from build123d import *

# Parameters (mm, degrees)
SKETCH6_W                    = 35
SKETCH6_H                    = 40
BASE_FLANGE2_DEPTH           = 1.4
EDGE_FLANGE1_STRIP_W         = 11.6
EDGE_FLANGE1_STRIP_H         = 1.4
EDGE_FLANGE1_STRIP_CUT_DEPTH = 40
EDGE_FLANGE1_DEPTH           = 40
EDGE_FLANGE2_STRIP_W         = 11.6
EDGE_FLANGE2_STRIP_H         = 1.4
EDGE_FLANGE2_STRIP_CUT_DEPTH = 40
EDGE_FLANGE2_DEPTH           = 40
EDGE_FLANGE3_STRIP_W         = 11.6
EDGE_FLANGE3_STRIP_H         = 1.4
EDGE_FLANGE3_STRIP_CUT_DEPTH = 40
EDGE_FLANGE3_DEPTH           = 40
EDGE_FLANGE4_STRIP_W         = 11.6
EDGE_FLANGE4_STRIP_H         = 1.4
EDGE_FLANGE4_STRIP_CUT_DEPTH = 40
EDGE_FLANGE4_DEPTH           = 40
CUT_EXTRUDE2_DEPTH           = 76.623541308
CUT_EXTRUDE2_DEPTH_BACK      = 76.623541308
SKETCH11_R                   = 7.5
SKETCH11_R_2                 = 1.7
CUT_EXTRUDE3_DEPTH           = 76.795514379
CUT_EXTRUDE3_DEPTH_BACK      = 76.795514379
SKETCH26_R                   = 1.7
CUT_EXTRUDE4_DEPTH           = 76.795514379
CUT_EXTRUDE4_DEPTH_BACK      = 76.795514379
SKETCH27_R                   = 1.7


# Sheet-metal steps are written as plain solids
with BuildPart() as part:
    # Sketch6 → Base-Flange2 (new body)
    with BuildSketch(Plane.XY):
        with Locations((17.5, 20)):
            Rectangle(SKETCH6_W, SKETCH6_H)
    extrude(amount=-BASE_FLANGE2_DEPTH)

    # Edge-Flange1 strip (across the edge) → Edge-Flange1 strip cut (cut)
    with BuildSketch(Plane.XZ.offset(-40)):
        with Locations((-1.4, -0.7)):
            Rectangle(EDGE_FLANGE1_STRIP_W, EDGE_FLANGE1_STRIP_H)
    extrude(amount=EDGE_FLANGE1_STRIP_CUT_DEPTH, mode=Mode.SUBTRACT)

    # Edge-Flange1 section (across the edge) → Edge-Flange1 (add)
    with BuildSketch(Plane.XZ.offset(-40)):
        with BuildLine():
            Line((0, 3), (0, 8.6))
            Line((0, 8.6), (1.4, 8.6))
            Line((1.4, 8.6), (1.4, 3))
            ThreePointArc((1.4, 3), (2.278679656, 0.878679656), (4.4, 0))
            Line((4.4, 0), (4.4, -1.4))
            ThreePointArc((4.4, -1.4), (1.288730163, -0.111269837), (0, 3))
        make_face()
    extrude(amount=EDGE_FLANGE1_DEPTH)

    # Edge-Flange2 strip (across the edge) → Edge-Flange2 strip cut (cut)
    with BuildSketch(Plane(origin=(35, 0, 0), x_dir=(-1, 0, 0), z_dir=(0, 1, 0))):
        with Locations((-1.4, -0.7)):
            Rectangle(EDGE_FLANGE2_STRIP_W, EDGE_FLANGE2_STRIP_H)
    extrude(amount=EDGE_FLANGE2_STRIP_CUT_DEPTH, mode=Mode.SUBTRACT)

    # Edge-Flange2 section (across the edge) → Edge-Flange2 (add)
    with BuildSketch(Plane(origin=(35, 0, 0), x_dir=(-1, 0, 0), z_dir=(0, 1, 0))):
        with BuildLine():
            Line((0, 3), (0, 8.6))
            Line((0, 8.6), (1.4, 8.6))
            Line((1.4, 8.6), (1.4, 3))
            ThreePointArc((1.4, 3), (2.278679656, 0.878679656), (4.4, 0))
            Line((4.4, 0), (4.4, -1.4))
            ThreePointArc((4.4, -1.4), (1.288730163, -0.111269837), (0, 3))
        make_face()
    extrude(amount=EDGE_FLANGE2_DEPTH)

    # Edge-Flange3 strip (across the edge) → Edge-Flange3 strip cut (cut)
    with BuildSketch(Plane(origin=(0, 0, 8.6), x_dir=(0, 0, -1), z_dir=(0, 1, 0))):
        with Locations((-1.4, -0.7)):
            Rectangle(EDGE_FLANGE3_STRIP_W, EDGE_FLANGE3_STRIP_H)
    extrude(amount=EDGE_FLANGE3_STRIP_CUT_DEPTH, mode=Mode.SUBTRACT)

    # Edge-Flange3 section (across the edge) → Edge-Flange3 (add)
    with BuildSketch(Plane(origin=(0, 0, 8.6), x_dir=(0, 0, -1), z_dir=(0, 1, 0))):
        with BuildLine():
            Line((0, 3), (0, 28.6))
            Line((0, 28.6), (1.4, 28.6))
            Line((1.4, 28.6), (1.4, 3))
            ThreePointArc((1.4, 3), (2.278679656, 0.878679656), (4.4, 0))
            Line((4.4, 0), (4.4, -1.4))
            ThreePointArc((4.4, -1.4), (1.288730163, -0.111269837), (0, 3))
        make_face()
    extrude(amount=EDGE_FLANGE3_DEPTH)

    # Edge-Flange4 strip (across the edge) → Edge-Flange4 strip cut (cut)
    with BuildSketch(Plane(origin=(35, 40, 8.6), x_dir=(0, 0, -1), z_dir=(0, -1, 0))):
        with Locations((-1.4, -0.7)):
            Rectangle(EDGE_FLANGE4_STRIP_W, EDGE_FLANGE4_STRIP_H)
    extrude(amount=EDGE_FLANGE4_STRIP_CUT_DEPTH, mode=Mode.SUBTRACT)

    # Edge-Flange4 section (across the edge) → Edge-Flange4 (add)
    with BuildSketch(Plane(origin=(35, 40, 8.6), x_dir=(0, 0, -1), z_dir=(0, -1, 0))):
        with BuildLine():
            Line((0, 3), (0, 28.6))
            Line((0, 28.6), (1.4, 28.6))
            Line((1.4, 28.6), (1.4, 3))
            ThreePointArc((1.4, 3), (2.278679656, 0.878679656), (4.4, 0))
            Line((4.4, 0), (4.4, -1.4))
            ThreePointArc((4.4, -1.4), (1.288730163, -0.111269837), (0, 3))
        make_face()
    extrude(amount=EDGE_FLANGE4_DEPTH)

    # Sketch11 → Cut-Extrude2 (cut, two sides: drawn at the far end of the back side and taken through both)
    with BuildSketch(Plane.XY.offset(-CUT_EXTRUDE2_DEPTH_BACK)):
        with Locations((17.5, 20)):
            Circle(SKETCH11_R)
        with Locations((17.5, 30)):
            Circle(SKETCH11_R_2)
        with Locations((8.839745962, 15)):
            Circle(SKETCH11_R_2)
        with Locations((26.160254038, 15)):
            Circle(SKETCH11_R_2)
    extrude(amount=CUT_EXTRUDE2_DEPTH + CUT_EXTRUDE2_DEPTH_BACK, mode=Mode.SUBTRACT)

    # Sketch26 → Cut-Extrude3 (cut, two sides: drawn at the far end of the back side and taken through both)
    with BuildSketch(Plane.XY.offset(8.6).offset(-CUT_EXTRUDE3_DEPTH_BACK)):
        with Locations(Location((-21.1, 35, 0), (0, 0, 180))):
            Circle(SKETCH26_R)
        with Locations(Location((-10.5, 35, 0), (0, 0, 180))):
            Circle(SKETCH26_R)
        with Locations(Location((-21.1, 5, 0), (0, 0, 180))):
            Circle(SKETCH26_R)
        with Locations(Location((-10.5, 5, 0), (0, 0, 180))):
            Circle(SKETCH26_R)
    extrude(amount=CUT_EXTRUDE3_DEPTH + CUT_EXTRUDE3_DEPTH_BACK, mode=Mode.SUBTRACT)

    # Sketch27 → Cut-Extrude4 (cut, two sides: drawn at the far end of the back side and taken through both)
    with BuildSketch(Plane.XY.offset(8.6).offset(-CUT_EXTRUDE4_DEPTH_BACK)):
        with Locations(Location((43, 35, 0), (0, 0, 180))):
            Circle(SKETCH27_R)
        with Locations(Location((58.6, 35, 0), (0, 0, 180))):
            Circle(SKETCH27_R)
        with Locations(Location((43, 5, 0), (0, 0, 180))):
            Circle(SKETCH27_R)
        with Locations(Location((58.6, 5, 0), (0, 0, 180))):
            Circle(SKETCH27_R)
    extrude(amount=CUT_EXTRUDE4_DEPTH + CUT_EXTRUDE4_DEPTH_BACK, mode=Mode.SUBTRACT)


solid = part.part
Design review of the part built by this model. Coordinates are the model's own, in mm. A direction names the side the tool comes from. Round coordinates to 2 decimals unless told otherwise and drop trailing zeros. Write each loop counter-clockwise with the first axis right and the second up, starting at its lowest first coordinate (ties: lowest second). Pieces come first, ordered by that corner, then holes. Notation, with made-up numbers: (-20, 30) - (-16, 30) arc R28 cw to (-16, 69) - close; hole circle Ø1 at (7, -9). An arc over 180 degrees is marked (long way). Use a Markdown table: item, result. Add a question column.
1. Wall thickness on probe 1 along Y at (x, z) = (43, 7.65); probe 2 along X at (y, z) = (38, 4); probe 3 along X at (y, z) = (15, -0.7): over which ranges is each line inside the solid? List them lowest first.
2. We need section B-B (x = -21.1). State the section outline as (y, z) points, then the cut area to 3 significant figures.
3. We need section C-C (y = 8.5). State the section outline as (x, z) points, then the cut area to 3 significant figures.
4. For faces 4 (the face through (2.26, 20.28, 0.9)), 5 (the face through (-11.3, 6.5, 7.9)), list the 3-axis set-ups (+Z, -Z, +X, -X, +Y, -Y) from which the entire face can be reached by the end or side of a thin tool; tool diameter is ignored.
5. Mouldability with a two-part tool opening along X and no side actions: class faces 1 (the face through (33.677, 19.72, -0.145)), 2 (the face through (24.46, 15.07, -0.71)), 3 (the face through (14.3, 0, -0.5)) as +X half, -X half, draft (parallel to the pull), parting line (faces both ways), or undercut.
6. We need section D-D (z = 6). State the section outline as (x, y) points, then the cut area to 3 significant figures.
7. We need section A-A (y = 20). State the section outline as (x, z) points.
8. Clearance check with flat-ended pins moving along their axes: pin 1 (3 mm diameter, centred on x = 24.5, y = 18, fed in from +Z); pin 2 (1 mm diameter, centred on y = 7.5, z = 5, fed in from +X); pin 3 (13 mm diameter, centred on x = -19.5, y = 19, fed in from -Z). State where each tip first meets the part, or that it passes through.
Output:
| question | item | result |
|---|---|---|
| 1 | probe 1 | y = 0 to 3.3, 6.7 to 33.3, 36.7 to 40 |
| 1 | probe 2 | x = 0 to 1.4, 33.6 to 35 |
| 1 | probe 3 | x = 2.02 to 7.14, 10.54 to 11.91, 23.09 to 24.46, 27.86 to 32.98 |
| 2 | outline | (0, 7.2) - (3.3, 7.2) - (3.3, 8.6) - (0, 8.6) - close; (6.7, 7.2) - (33.3, 7.2) - (33.3, 8.6) - (6.7, 8.6) - close; (36.7, 7.2) - (40, 7.2) - (40, 8.6) - (36.7, 8.6) - close |
| 2 | area | 46.5 mm2 |
| 3 | outline | (-28.6, 7.2) - (-3, 7.2) arc R3 cw to (0, 4.2) - (0, 3) arc R4.4 ccw to (4.4, -1.4) - (30.6, -1.4) arc R4.4 ccw to (35, 3) - (35, 4.2) arc R3 cw to (38, 7.2) - (63.6, 7.2) - (63.6, 8.6) - (38, 8.6) arc R4.4 ccw to (33.6, 4.2) - (33.6, 3) arc R3 cw to (30.6, 0) - (4.4, 0) arc R3 cw to (1.4, 3) - (1.4, 4.2) arc R4.4 ccw to (-3, 8.6) - (-28.6, 8.6) - close |
| 3 | area | 144 mm2 |
| 4 | face 4 | +Z, +Y, -Y |
| 4 | face 5 | +Z, -Z |
| 5 | face 1 | +X half |
| 5 | face 2 | undercut |
| 5 | face 3 | draft |
| 6 | outline | (-0.6, 0) - (1.01, 0) - (1.01, 40) - (-0.6, 40) - close; (33.99, 0) - (35.6, 0) - (35.6, 40) - (33.99, 40) - close |
| 6 | area | 129 mm2 |
| 7 | outline | (-28.6, 7.2) - (-3, 7.2) arc R3 cw to (0, 4.2) - (0, 3) arc R4.4 ccw to (4.4, -1.4) - (10, -1.4) - (10, 0) - (4.4, 0) arc R3 cw to (1.4, 3) - (1.4, 4.2) arc R4.4 ccw to (-3, 8.6) - (-28.6, 8.6) - close; (25, -1.4) - (30.6, -1.4) arc R4.4 ccw to (35, 3) - (35, 4.2) arc R3 cw to (38, 7.2) - (63.6, 7.2) - (63.6, 8.6) - (38, 8.6) arc R4.4 ccw to (33.6, 4.2) - (33.6, 3) arc R3 cw to (30.6, 0) - (25, 0) - close |
| 8 | pin 1 | stops at z = 0 |
| 8 | pin 2 | stops at x = 35.3 |
| 8 | pin 3 | stops at z = 7.2 |
